Model file for the job. Use its own axes, mm. A direction names the side the tool comes from. Give positions to 0.01 mm unless a question says otherwise; leave off trailing zeros. Order: outer loops, then holes, each group sorted by start corner. A loop starts at its lowest first (then second) coordinate and runs counter-clockwise, first axis right, second up. Notation, with made-up numbers: (17, 29.25) -> (59, 29.25) arc R5 ccw to (59, 33.25) -> close; hole circle Ø4 at (38.5, -23.75). An arc over 180 degrees is marked (long way). Answer in a Markdown table with one row per item. Add a question column.
from build123d import *

# Parameters (mm, degrees)
SKETCH_1_R      = 0.9
EXTRUDE_1_DEPTH = 2


with BuildPart() as part:
    # 草图1 → 凸台-拉伸1 (new body)
    with BuildSketch(Plane.XY):
        with BuildLine():
            Line((-13.95, -5.299998555), (-13.95, -6.75))
            Line((-13.95, -6.75), (-10.95, -6.75))
            ThreePointArc((-10.95, -6.75), (-5.506483958, -5.47673518), (-0.23016259, -7.324301965))
            ThreePointArc((-0.23016259, -7.324301965), (2.253977211, -8.570843532), (5, -9))
            ThreePointArc((5, -9), (7.25, -6.75), (5, -4.5))
            ThreePointArc((5, -4.5), (0.5, 0), (5, 4.5))
            ThreePointArc((5, 4.5), (7.25, 6.75), (5, 9))
            ThreePointArc((5, 9), (2.253977211, 8.570843532), (-0.23016259, 7.324301965))
            ThreePointArc((-0.23016259, 7.324301965), (-5.506483958, 5.47673518), (-10.95, 6.75))
            Line((-10.95, 6.75), (-13.95, 6.75))
            Line((-13.95, 6.75), (-13.95, 5.299998555))
            ThreePointArc((-13.95, 5.299998555), (-13.737867966, 4.787866521), (-14.25, 4.999998555))
            Line((-14.25, 4.999998555), (-15.75, 4.999998555))
            ThreePointArc((-15.75, 4.999998555), (-16.262132034, 4.787866521), (-16.05, 5.299998555))
            Line((-16.05, 5.299998555), (-16.05, 6.75))
            Line((-16.05, 6.75), (-18.05, 6.75))
            Line((-18.05, 6.75), (-18.05, -6.75))
            Line((-18.05, -6.75), (-16.05, -6.75))
            Line((-16.05, -6.75), (-16.05, -5.299998555))
            ThreePointArc((-16.05, -5.299998555), (-16.262132034, -4.787866521), (-15.75, -4.999998555))
            Line((-15.75, -4.999998555), (-14.25, -4.999998555))
            ThreePointArc((-14.25, -4.999998555), (-13.737867966, -4.787866521), (-13.95, -5.299998555))
        make_face()
        with Locations((-6, 0)):
            Circle(SKETCH_1_R, mode=Mode.SUBTRACT)
        with Locations((5, 6.75)):
            Circle(SKETCH_1_R, mode=Mode.SUBTRACT)
        with Locations((5, -6.75)):
            Circle(SKETCH_1_R, mode=Mode.SUBTRACT)
    extrude(amount=EXTRUDE_1_DEPTH)


solid = part.part
Item 1: Two-plate mould, pull along X, no slides. Class faces 5 (the cylindrical face through (7.25, 6.7, 0.99)), 6 (the flat face through (-17, 6.75, 1)), 7 (the cylindrical face through (-5.586, -5.473, 0.986)): pulls with the +X half, pulls with the -X half, needs draft (parallel to the pull), parting line crosses it, or undercut.
Item 2: Pin check, flat tips, straight feed: pin 1 Ø0.8 at (x, z) = (-14.5, 0.5) entering from +Y; pin 2 Ø0.5 at (x, z) = (-15.5, 1.5) entering from -Y; pin 3 Ø0.7 at (y, z) = (6, 1) entering from +X; pin 4 Ø1.4 at (x, y) = (5, -6.75) entering from -Z. Stop position of each tip, or through.
Item 3: Wall check: line 1 (Y direction, x = -14.75, z = 0.6); line 2 (Y direction, x = -12.25, z = 0.25); line 3 (X direction, y = 5.25, z = 0.1). Give the ranges that are in metal, low to high.
Item 4: Which spindle directions (+Z, -Z, +X, -X, +Y, -Y) get a long thin tool onto all of the face, cutting with end or side? Do faces 1 (the flat face through (-17, -6.75, 1)), 2 (the flat face through (-12, 6.75, 1)), 3 (the flat face through (-16.05, -6, 1)), 4 (the flat face through (-15, 5, 1)). Say none if no direction does.
Item 5: Saw through at B-B on y = 0. List the corners of the cut face in (x, z), plus the area to 3 significant figures.
Item 6: Saw through at C-C on x = -6. List the corners of the cut face in (y, z), plus the area to 4 significant figures.
Item 7: Saw through at D-D on x = -11.25. List the corners of the cut face in (y, z), plus the area to 3 significant figures.
Item 8: Saw through at A-A on z = 0.7. List the corners of the cut face in (x, y), plus the area to 3 significant figures.
Evaluation:
| question | item | result |
|---|---|---|
| 1 | face 5 | pulls with the +X half |
| 1 | face 6 | needs draft |
| 1 | face 7 | undercut |
| 2 | pin 1 | stops at y = 5 |
| 2 | pin 2 | stops at y = -5 |
| 2 | pin 3 | stops at x = 7.21 |
| 2 | pin 4 | passes through |
| 3 | line 1 | y = -5 to 5 |
| 3 | line 2 | y = -6.75 to 6.75 |
| 3 | line 3 | x = -18.05 to -16.22, -13.78 to 6.68 |
| 4 | face 1 | +Z, -Z, -X, -Y |
| 4 | face 2 | +Z, -Z, -X, +Y |
| 4 | face 3 | +Z, -Z, -Y |
| 4 | face 4 | +Z, -Z, +Y |
| 5 | outline | (-18.05, 0) -> (-6.9, 0) -> (-6.9, 2) -> (-18.05, 2) -> close; (-5.1, 0) -> (0.5, 0) -> (0.5, 2) -> (-5.1, 2) -> close |
| 5 | area | 33.5 mm2 |
| 6 | outline | (-5.46, 0) -> (-0.9, 0) -> (-0.9, 2) -> (-5.46, 2) -> close; (0.9, 0) -> (5.46, 0) -> (5.46, 2) -> (0.9, 2) -> close |
| 6 | area | 18.25 mm2 |
| 7 | outline | (-6.75, 0) -> (6.75, 0) -> (6.75, 2) -> (-6.75, 2) -> close |
| 7 | area | 27.0 mm2 |
| 8 | outline | (-18.05, -6.75) -> (-16.05, -6.75) -> (-16.05, -5.3) arc R0.3 cw (long way) to (-15.75, -5) -> (-14.25, -5) arc R0.3 cw (long way) to (-13.95, -5.3) -> (-13.95, -6.75) -> (-10.95, -6.75) arc R10 cw to (-0.23, -7.32) arc R9 ccw to (5, -9) arc R2.25 ccw to (5, -4.5) arc R4.5 cw to (5, 4.5) arc R2.25 ccw to (5, 9) arc R9 ccw to (-0.23, 7.32) arc R10 cw to (-10.95, 6.75) -> (-13.95, 6.75) -> (-13.95, 5.3) arc R0.3 cw (long way) to (-14.25, 5) -> (-15.75, 5) arc R0.3 cw (long way) to (-16.05, 5.3) -> (-16.05, 6.75) -> (-18.05, 6.75) -> close; hole circle Ø1.8 at (-6, 0); hole circle Ø1.8 at (5, -6.75); hole circle Ø1.8 at (5, 6.75) |
| 8 | area | 281 mm2 |
